from build123d import *

# Parameters (mm, degrees)
SKETCH2_R               = 44.45
SKETCH2_W               = 5.461
SKETCH2_H               = 25.4
BOSS_EXTRUDE1_DEPTH     = 5.588
SKETCH3_R               = 3.175
CUT_EXTRUDE1_DEPTH      = 64.109672349
FILL_PATTERN1_OUTLINE_R = 3.175
FILL_PATTERN1_DEPTH     = 5.588


# Read off the part's stored shape, not the designer's step: Fill Pattern1
with BuildPart() as part:
    # Sketch2 → Boss-Extrude1 (new body)
    with BuildSketch(Plane(origin=(0, 0, 0), x_dir=(1, 0, 0), z_dir=(0, 1, 0))):
        with Locations(Location((0, 0, 0), (0, 0, 270))):
            Circle(SKETCH2_R)
        with Locations((0, 25.4)):
            Rectangle(SKETCH2_W, SKETCH2_H, mode=Mode.SUBTRACT)
        Polygon((34.360817884, -16.685317635), (31.630317884, -21.414682365), (9.633272628, -8.714682365), (12.363772628, -3.985317635), align=None, mode=Mode.SUBTRACT)
        Polygon((-31.630317884, -21.414682365), (-34.360817884, -16.685317635), (-12.363772628, -3.985317635), (-9.633272628, -8.714682365), align=None, mode=Mode.SUBTRACT)
    extrude(amount=BOSS_EXTRUDE1_DEPTH)

    # Sketch3 → Cut-Extrude1 (cut, through all)
    with BuildSketch(Plane(origin=(0, 5.588, 0), x_dir=(1, 0, 0), z_dir=(0, 1, 0))):
        with Locations(Location((0, 0, 0), (0, 0, 270))):
            Circle(SKETCH3_R)
    extrude(amount=-CUT_EXTRUDE1_DEPTH, mode=Mode.SUBTRACT)

    # Fill Pattern1 outline → Fill Pattern1 (cut)
    with BuildSketch(Plane(origin=(0, 0, 0), x_dir=(1, 0, 0), z_dir=(0, 1, 0))):
        with Locations((34.697045256, 9.297045256)):
            Circle(FILL_PATTERN1_OUTLINE_R)
        with Locations((9.297045256, -34.697045256)):
            Circle(FILL_PATTERN1_OUTLINE_R)
        with Locations((-12.7, -21.997045256)):
            Circle(FILL_PATTERN1_OUTLINE_R)
        with Locations((-34.697045256, -9.297045256)):
            Circle(FILL_PATTERN1_OUTLINE_R)
        with Locations((-21.997045256, 12.7)):
            Circle(FILL_PATTERN1_OUTLINE_R)
        with Locations((-9.297045256, 34.697045256)):
            Circle(FILL_PATTERN1_OUTLINE_R)
        with Locations((12.7, 21.997045256)):
            Circle(FILL_PATTERN1_OUTLINE_R)
    extrude(amount=FILL_PATTERN1_DEPTH, mode=Mode.SUBTRACT)


solid = part.part
Build history of the part. All positions in model axes, mm. Round coordinates to 2 decimals unless told otherwise and drop trailing zeros. Write each loop counter-clockwise with the first axis right and the second up, starting at its lowest first coordinate (ties: lowest second). Pieces come first, ordered by that corner, then holes. Notation, with made-up numbers: (45, 72.5) -> (86, 72.5) arc R25 ccw to (86, 105.5) -> close; hole circle Ø6 at (23, -12.75). An arc over 180 degrees is marked (long way). Write item = value, one per line.
(1) Band-saw the part on A-A (z = 0). Give the cut face in (x, y) (3 decimals), then the cut area to 3 significant figures.
Answer:
outline = (-44.45, 0) -> (-3.175, 0) -> (-3.175, 5.588) -> (-44.45, 5.588) -> close; (3.175, 0) -> (44.45, 0) -> (44.45, 5.588) -> (3.175, 5.588) -> close
area = 461 mm2
(2) Probe L1, parallel to Z at x = -20.5, y = 3.9; L2, parallel to X at y = 4.7, z = -14; L3, parallel to X at y = 0.3, z = -33.5. List the from-to ranges inside material, lowest first.
Answer:
L1 = -39.44 to -15.5, -9.9 to 8.68, 14.99 to 39.44
L2 = -42.19 to -24.89, -19.1 to -2.73, 2.73 to 42.19
L3 = -29.22 to -12.24, -6.36 to -2.73, 2.73 to 29.22
(3) Flat gauge pins, fed straight in: pin 1 (7.5 mm diameter, centred on x = 0, z = 0, fed in from +Y); pin 2 (3 mm diameter, centred on x = -33, y = 4, fed in from +Z); pin 3 (3 mm diameter, centred on y = 1, z = -27.5, fed in from -X); pin 4 (3 mm diameter, centred on y = 3, z = 25, fed in from +X). Where does each tip first touch, or does it go through?
Answer:
pin_1 = 5.59
pin_2 = 31.36
pin_3 = -36.05
pin_4 = 37.73
(4) Band-saw the part on B-B (x = 19.5). Give the cut face in (y, z).
Answer:
outline = (0, -39.94) -> (5.59, -39.94) -> (5.59, 8.11) -> (0, 8.11) -> close; (0, 14.41) -> (5.59, 14.41) -> (5.59, 39.94) -> (0, 39.94) -> close
(5) Band-saw the part on C-C (y = 1.2). State how many separate pieces and enclosed holes the cut face has, then the cut area to 3 significant figures.
Answer:
separate_pieces = 1
enclosed_holes = 11
area = 5,540 mm2
(6) Two-plate mould, pull along X, no slides. Class faces 1 (the face through (-9, 5.588, -1)), 2 (the face through (-1.93, 2.83, -2.52)), 3 (the face through (23.208, 2.755, 10.246)), 4 (the face through (37.48, 2.75, 23.9)): pulls with the +X half, pulls with the -X half, needs draft (parallel to the pull), parting line crosses it, or undercut.
Answer:
face_1 = needs draft
face_2 = undercut
face_3 = undercut
face_4 = parting line crosses it
(7) Band-saw the part on D-D (x = -11). Give the cut face in (y, z), then the cut area to 3 significant figures.
Answer:
outline = (0, -43.07) -> (5.59, -43.07) -> (5.59, -37.38) -> (0, -37.38) -> close; (0, -32.02) -> (5.59, -32.02) -> (5.59, 6.35) -> (0, 6.35) -> close; (0, 9.5) -> (5.59, 9.5) -> (5.59, 19.32) -> (0, 19.32) -> close; (0, 24.68) -> (5.59, 24.68) -> (5.59, 43.07) -> (0, 43.07) -> close
area = 404 mm2
